from build123d import *

# Parameters (mm, degrees)
F1_DEPTH  = 12.7
F2_DEPTH  = 2.54
F3_DEPTH  = 7.62
F4_DEPTH  = 2.54
F5_DEPTH  = 2.54
F6_DEPTH  = 2.54
F7_DEPTH  = 2.54
F8_DEPTH  = 2.54
F9_DEPTH  = 2.54
F10_R     = 16.050678096
F10_R_2   = 13.472274859
F10_R_3   = 3.0244847624
F10_R_4   = 2.9484981223
F10_R_5   = 2.9899979454
F11_DEPTH = 10.16


with BuildPart() as f1:
    # F0 (on Front) → F1 (new body)
    with BuildSketch(Plane.XZ):
        Polygon((59.2296272516, 26.558874175), (0, 68.5641244054), (-54.7846257687, 26.558874175), (-54.7846257687, -40.5606217682), (0, -72.7868750691), (59.2296272516, -40.5606217682), align=None)
    extrude(amount=F1_DEPTH)

    # F2 (cut): a face of the model
    f2_faces = [f1.faces().sort_by_distance(p)[0] for p in [
        (1.9587071028, -12.7, -4.2659517496),
    ]]
    extrude(f2_faces, amount=-F2_DEPTH, mode=Mode.SUBTRACT)

    # F3 (cut): a face of the model
    f3_faces = [f1.faces().sort_by_distance(p)[0] for p in [
        (1.9587071028, -10.16, -4.2659517496),
    ]]
    extrude(f3_faces, amount=-F3_DEPTH, mode=Mode.SUBTRACT)

    # F4 (cut): a face of the model
    f4_faces = [f1.faces().sort_by_distance(p)[0] for p in [
        (29.6148136258, -1.27, 47.5614992902),
    ]]
    extrude(f4_faces, amount=-F4_DEPTH, mode=Mode.SUBTRACT)

    # F5 (cut): a face of the model
    f5_faces = [f1.faces().sort_by_distance(p)[0] for p in [
        (-27.3923128843, -1.27, 47.5614992902),
    ]]
    extrude(f5_faces, amount=-F5_DEPTH, mode=Mode.SUBTRACT)

    # F6 (cut): a face of the model
    f6_faces = [f1.faces().sort_by_distance(p)[0] for p in [
        (59.2296272516, -1.27, -7.0008737966),
    ]]
    extrude(f6_faces, amount=-F6_DEPTH, mode=Mode.SUBTRACT)

    # F7 (cut): a face of the model
    f7_faces = [f1.faces().sort_by_distance(p)[0] for p in [
        (-54.7846257687, -1.27, -7.0008737966),
    ]]
    extrude(f7_faces, amount=-F7_DEPTH, mode=Mode.SUBTRACT)

    # F8 (cut): a face of the model
    f8_faces = [f1.faces().sort_by_distance(p)[0] for p in [
        (-27.3923128843, -1.27, -56.6737484187),
    ]]
    extrude(f8_faces, amount=-F8_DEPTH, mode=Mode.SUBTRACT)

    # F9 (cut): a face of the model
    f9_faces = [f1.faces().sort_by_distance(p)[0] for p in [
        (29.6148136258, -1.27, -56.6737484187),
    ]]
    extrude(f9_faces, amount=-F9_DEPTH, mode=Mode.SUBTRACT)

    # F10 (on face) → F11 (join)
    with BuildSketch(Plane.XZ.offset(2.54)):
        with Locations((-32.0333689451, -24.9490719289)):
            Circle(F10_R)
        with Locations((-32.0333689451, -24.9490719289)):
            Circle(F10_R_2, mode=Mode.SUBTRACT)
        with Locations((-32.0333689451, -17.3833221197)):
            Circle(F10_R_3)
        with Locations((-25.150520727, -28.8595743477)):
            Circle(F10_R_4)
        with Locations((-38.8115644455, -28.9213098586)):
            Circle(F10_R_5)
        Polygon((-26.3045579195, -21.8257736415), (-37.7313010395, -21.8257736415), (-31.9700799882, -31.7595750093), align=None)
    extrude(amount=F11_DEPTH)


solid = f1.part
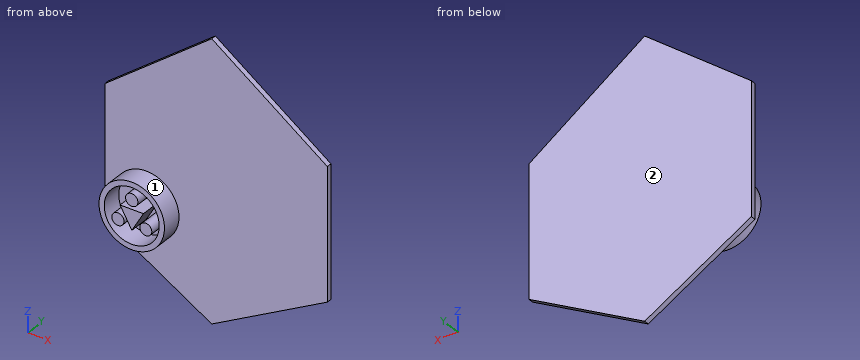
Can you work these out from the model? Positions are in its coordinate system, mm. Face numbers are marked on the shaded views. A direction names the side the tool comes from. Round coordinates to 2 decimals unless told otherwise and drop trailing zeros. Order: outer loops, then holes, each group sorted by start corner. A loop starts at its lowest first (then second) coordinate and runs counter-clockwise, first axis right, second up. Notation, with made-up numbers: M 31,48.25 L 55,48.25 A30 ccw 55,87.25 Z; hole C -16,54.5 d5. An arc over 180 degrees is marked long. Use a Markdown table: item, result.
1) If I drill on line 1 along X through (y, z) = (-8.5, -19); line 2 along Z through (x, y) = (-32, -10.5); line 3 along Y through (x, z) = (2.5, 40), over which ranges is the centre line in solid material (lowest first)?
Geometry says:
| item | result |
|---|---|
| line 1 | x = -46.94 to -44.12, -34.59 to -29.48, -19.95 to -17.13 |
| line 2 | z = -41 to -38.42, -31.71 to -21.83, -20.41 to -14.36, -11.48 to -8.9 |
| line 3 | y = -2.54 to 0 |
2) On a 3-axis mill with a long thin cutter (end or side, diameter ignored), from which of +Z, -Z, +X, -X, +Y, -Y can I reach the whole of each face in a straight line? I mean the marked faces 1 and 2. Say none if no direction works.
Geometry says:
| item | result |
|---|---|
| face 1 | -Y |
| face 2 | +Z, -Z, +X, -X, +Y |
3) Imagine slicing it at A-A (y = -9.5). List the corners of the cut face in (x, z) for me.
Geometry says:
| item | result |
|---|---|
| outline | C -32.03,-24.95 d32.1; C -38.81,-28.92 d5.98; M -37.73,-21.83 L -31.97,-31.76 L -26.3,-21.83 Z; C -32.03,-17.38 d6.05; C -25.15,-28.86 d5.9; hole C -32.03,-24.95 d26.94 |
4) I'm going to push flat-ended pins straight in: P1, Ø3, axis at x = -31, y = -10, coming from the +Z side; P2, Ø3, axis at x = -25.5, y = -8, coming from the -Z side. Where does each tip first touch, or does it pass through?
Geometry says:
| item | result |
|---|---|
| P1 | stops at z = -8.9 |
| P2 | stops at z = -40.19 |
5) Imagine slicing it at B-B (z = -5.5). List the corners of the cut face in (x, y) for me, then the cut area to 3 significant figures.
Geometry says:
| item | result |
|---|---|
| outline | M -52.24,-2.54 L 56.69,-2.54 L 56.69,0 L -52.24,0 Z |
| area | 277 mm² |
6) Imagine slicing it at C-C (x = 21). List the corners of the cut face in (y, z) for me.
Geometry says:
| item | result |
|---|---|
| outline | M -2.54,-58.47 L 0,-58.47 L 0,50.56 L -2.54,50.56 Z |
